Input: part model. Units: mm. Frame: model coordinates. A direction names the side the tool comes from. Coordinates: 2 decimals unless noted, no trailing zeros. Loops run counter-clockwise (first coordinate to the right, second up) from the corner with the lowest first, then second, coordinate; pieces in that order, holes last. Notation, with made-up numbers: (20.5, 82) -> (57.5, 82) arc R18 cw to (57.5, 93) -> close; hole circle Ø6 at (37.25, 82). An arc over 180 degrees is marked (long way). Put each result on its own line as item: value. Start each with the question number.
1) Cut plane C-C (y = 29.37). Return the cut outline in (x, z) (3 decimals).
2) Contact query for flat-ended pins moving along their axis: P1, Ø24, axis at x = 5.5, y = 27, coming from the +Z side; P2, Ø6.5, axis at x = 4, y = 31, coming from the -Z side; P3, Ø0.5, axis at x = -3.5, z = 12.5, coming from the +Y side. Output: stop coordinate, or through.
3) Cut plane D-D (x = -16.5). State how many separate pieces and enclosed holes the cut face has, plus the area to 3 significant figures.
4) Material intervals for L1, parallel to Y at x = 0, z = 3.4; L2, parallel to Y at x = 15.37, z = 6; L3, parallel to X at y = 15, z = 5.75, sorted ascending.
5) Pull-direction query (X, two-part tool) for faces 4 (the cylindrical face through (21.4, 59.43, 4.06)), 5 (the cylindrical face through (1.45, 40.45, 2.46)), 6 (the cylindrical face through (-2.54, 33.354, 6.479)), 7 (the flat face through (0, 4, 13)); classes: pulls with the +X half, pulls with the -X half, needs draft (parallel to the pull), parting line crosses it, or undercut.
6) Set-up query: faces 1 (the flat face through (11, 24, 0)), 2 (the flat face through (0, 35, 8)), 3 (the flat face through (-5, 30, 5)). Return all of +Z, -Z, +X, -X, +Y, -Y with unobstructed straight access to the full face (end or side cutting, diameter ignored); none if empty.
7) Cut plane A-A (y = 15.5). Return the cut outline in (x, z), plus the area to 3 significant figures.
8) Cut plane B-B (z = 2.5). Return the cut outline in (x, y).
from build123d import *

# Parameters (mm, degrees)
BOSS_EXTRUDE1_DEPTH  = 8
BOSS_EXTRUDE2_DEPTH  = 5
SKETCH3_R            = 1.5
CUT_EXTRUDE_DEPTH    = 8
FILLET1_SIZE         = 2
FILLET1_SIZE_2       = 4
FILLET2_R            = 2
SKETCH4_R            = 4.0005
SKETCH4_R_2          = 4.725
M4_H6_T_INSERT_DEPTH = 8
SKETCH13_R           = 11.176
CUT_EXTRUDE2_DEPTH   = 5
SKETCH14_R           = 2.6
CUT_EXTRUDE3_DEPTH   = 67.287253734


with BuildPart() as part:
    # Sketch1 → Boss-Extrude1 (new body)
    with BuildSketch(Plane.XY):
        with BuildLine():
            Line((22, 60), (-22, 60))
            ThreePointArc((-22, 60), (-22.750468165, 29.962523408), (-25, 0))
            Line((-25, 0), (25, 0))
            ThreePointArc((25, 0), (22.750468165, 29.962523408), (22, 60))
        make_face()
    extrude(amount=BOSS_EXTRUDE1_DEPTH)

    # Sketch2 → Boss-Extrude2 (add)
    with BuildSketch(Plane.XY.offset(8)):
        with BuildLine():
            Line((-25, 0), (25, 0))
            ThreePointArc((25, 0), (24.612606496, 3.998750886), (24.251929498, 8))
            Line((24.251929498, 8), (-24.251929498, 8))
            ThreePointArc((-24.251929498, 8), (-24.612606496, 3.998750886), (-25, 0))
        make_face()
    extrude(amount=BOSS_EXTRUDE2_DEPTH)

    # Sketch3 → Cut-Extrude (cut)
    with BuildSketch(Plane(origin=(0, 8, 0), x_dir=(1, 0, 0), z_dir=(0, 1, 0))):
        with Locations(Location((-19.251929498, -10.5, 0), (0, 0, 270))):
            Circle(SKETCH3_R)
        with Locations(Location((19.251929498, -10.5, 0), (0, 0, 270))):
            Circle(SKETCH3_R)
    extrude(amount=-CUT_EXTRUDE_DEPTH, mode=Mode.SUBTRACT)

    # Fillet1
    # an asymmetric fillet: 4, 2 mm, written as the material it adds along each edge
    with BuildSketch(Plane(origin=(34.251929498, 8, 8), x_dir=(0, 1, 0), z_dir=(-1, 0, 0))) as fillet1_piece_1_section:
        with BuildLine():
            Bezier((FILLET1_SIZE, 0), (0, 0), (0, -FILLET1_SIZE_2), weights=[1, 0.707106781, 1])
            Line((0, -FILLET1_SIZE_2), (-0.08, -4))
            Line((-0.08, -4), (-0.08, 0.08))
            Line((-0.08, 0.08), (2, 0.08))
            Line((2, 0.08), (FILLET1_SIZE, 0))
        make_face()
    fillet1_piece_1 = extrude(amount=68.503858997, mode=Mode.PRIVATE)
    fillet1_piece_1 = fillet1_piece_1 - Plane(origin=(-623.5, 60, 8.94437244), x_dir=(1, 0, 0), z_dir=(0, 0, -1)) * Cylinder(601.5, 154, mode=Mode.PRIVATE)
    fillet1_piece_1 = fillet1_piece_1 - Plane(origin=(623.5, 60, 8.94437244), x_dir=(-0.9950124688279272, -0.09975062344142714, 0), z_dir=(0, 0, -1)) * Cylinder(601.5, 154, mode=Mode.PRIVATE)
    fillet1_piece_1 = fillet1_piece_1 - Plane(origin=(-19.251929498, 8.425610742, 10.5), x_dir=(0, 0, 1), z_dir=(0, 1, 0)) * Cylinder(1.5, 154, mode=Mode.PRIVATE)
    fillet1_piece_1 = fillet1_piece_1 - Plane(origin=(19.251929498, 8.425610742, 10.5), x_dir=(0, 0, 1), z_dir=(0, 1, 0)) * Cylinder(1.5, 154, mode=Mode.PRIVATE)
    add(fillet1_piece_1)

    # Fillet2
    fillet2_edges = [part.edges().sort_by_distance(p)[0] for p in [
        (22, 60, 4),
        (-22, 60, 4),
    ]]
    fillet(fillet2_edges, radius=FILLET2_R)

    # Sketch4 → M4*H6 T-Insert (cut)
    with BuildSketch(Plane(origin=(0, 0, 0), x_dir=(-1, 0, 0), z_dir=(0, 0, -1))):
        with Locations((0, 52)):
            Circle(SKETCH4_R)
        with Locations((0, 29.37)):
            Circle(SKETCH4_R_2)
    extrude(amount=-M4_H6_T_INSERT_DEPTH, mode=Mode.SUBTRACT)

    # Sketch13 → Cut-Extrude2 (cut)
    with BuildSketch(Plane(origin=(0, 0, 0), x_dir=(-1, 0, 0), z_dir=(0, 0, -1))):
        with Locations((0, 29.37)):
            Circle(SKETCH13_R)
    extrude(amount=-CUT_EXTRUDE2_DEPTH, mode=Mode.SUBTRACT)

    # Sketch14 → Cut-Extrude3 (cut, through all)
    with BuildSketch(Plane(origin=(0, 0, 0), x_dir=(-1, 0, 0), z_dir=(0, 0, -1))):
        with Locations((15.364, 14.003)):
            Circle(SKETCH14_R)
        with Locations((15.364, 44.737)):
            Circle(SKETCH14_R)
        with Locations((-15.37, 44.737)):
            Circle(SKETCH14_R)
        with Locations((-15.37, 14.003)):
            Circle(SKETCH14_R)
    extrude(amount=-CUT_EXTRUDE3_DEPTH, mode=Mode.SUBTRACT)


solid = part.part
Results found:
1. outline: (-22.78, 0) -> (-11.176, 0) -> (-11.176, 5) -> (-4.725, 5) -> (-4.725, 8) -> (-22.78, 8) -> close; (4.725, 5) -> (11.176, 5) -> (11.176, 0) -> (22.78, 0) -> (22.78, 8) -> (4.725, 8) -> close
2. P1: stops at z = 8
2. P2: stops at z = 5
2. P3: stops at y = 8
3. separate pieces: 3
3. enclosed holes: 0
3. area: 447 mm2
4. L1: y = 0 to 18.19, 40.55 to 48, 56 to 60
4. L2: y = 0 to 11.4, 16.6 to 42.14, 47.34 to 60
4. L3: x = -23.69 to -17.77, -12.96 to 12.97, 17.77 to 23.69
5. face 4: pulls with the +X half
5. face 5: undercut
5. face 6: undercut
5. face 7: needs draft
6. face 1: -Z, +X, -X, +Y, -Y
6. face 2: +Z, +X, -X, +Y
6. face 3: -Z
7. outline: (-23.65, 0) -> (-17.49, 0) -> (-17.49, 8) -> (-23.65, 8) -> close; (-13.24, 0) -> (13.24, 0) -> (13.24, 8) -> (-13.24, 8) -> close; (17.5, 0) -> (23.65, 0) -> (23.65, 8) -> (17.5, 8) -> close
7. area: 310 mm2
8. outline: (-25, 0) -> (25, 0) arc R601.5 cw to (22, 58.01) arc R2 ccw to (20, 60) -> (-20, 60) arc R2 ccw to (-22, 58.01) arc R601.5 cw to start; hole circle Ø5.2 at (-15.36, 14); hole circle Ø5.2 at (-15.36, 44.74); hole circle Ø22.35 at (0, 29.37); hole circle Ø8 at (0, 52); hole circle Ø5.2 at (15.37, 14); hole circle Ø5.2 at (15.37, 44.74)
